Build history of the part. All positions in model axes, mm. A direction names the side the tool comes from. Coordinates: 2 decimals unless noted, no trailing zeros. Loops run counter-clockwise (first coordinate to the right, second up) from the corner with the lowest first, then second, coordinate; pieces in that order, holes last.
(1) Wall check: L1, parallel to Y at x = -120, z = 8.25; L2, parallel to X at y = -18, z = 8.5; L3, parallel to X at y = -18.5, z = 6.5. Give the ranges that are in metal, low to high.
(2) Slice it at D-D (x = 73). Give the cut face in (y, z), and give its area (3 significant figures).
(3) Slice it at B-B (z = 7). Give the number of separate pieces and of enclosed holes in the cut face, and give its area (3 significant figures).
(4) Flat gauge pins, fed straight in: P1, Ø5, axis at x = -32.04, y = -18.5, coming from the -Z side; P2, Ø1.9, axis at x = -97.09, y = 54.66, coming from the +Z side. Where does each tip first touch, or does it go through?
(5) Slice it at C-C (x = -49.5). Give the cut face in (y, z).
(6) Slice it at A-A (x = 8.5). Give the cut face in (y, z).
(7) Two-plate mould, pull along X, no slides. Class faces 1 (the face through (-150, -2, 5)), 2 (the face through (2, -150, 5)), 3 (the face through (1, -39, 3)): pulls with the +X half, pulls with the -X half, needs draft (parallel to the pull), parting line crosses it, or undercut.
(8) Tool access for faces 4 (the face through (-41.53, -79.845, 1.479)), 5 (the face through (-2, 150, 5)): list every direction of +Z, -Z, +X, -X, +Y, -Y with a clear straight run to the whole face (end or side of a thin tool).
Autodesk Inventor part; units mm, degrees
ref_plane "YZ Plane" through (0, 0, 0) normal (1, 0, 0) x (0, 1, 0)
ref_plane "XZ Plane" through (0, 0, 0) normal (0, 1, 0) x (-1, 0, 0)
ref_plane "XY Plane" through (0, 0, 0) normal (0, 0, 1) x (1, 0, 0)
sketch "スケッチ1" plane through (-150, -150, 0) normal (0, 0, 1) x (1, 0, 0)
  circle A0 centre (59.9853, 240.0147) radius 24 construction
  circle A1 centre (59.9853, 240.0147) radius 24 construction
  circle A2 centre (84.0269, 264.0563) radius 10 construction
  line L0 (84.0269, 264.0563) -> (59.9853, 240.0147) construction
  line L1 (59.9853, 240.0147) -> (84.0269, 215.9731) construction
  arc A3 (84.5273, 253.0677) -> (73.0383, 264.5567) centre (84.0269, 264.0563) ccw
  arc A4 (70.2215, 262.823) -> (82.7936, 250.2509) centre (59.9853, 240.0147) ccw
  arc A5 (84.5273, 253.0677) -> (82.7936, 250.2509) centre (84.6183, 251.0698) ccw
  arc A6 (70.2215, 262.823) -> (73.0383, 264.5567) centre (71.0404, 264.6477) ccw
  line L2 (67.0564, 275.37) -> (24.63, 232.9436) construction
  line L3 (24.63, 232.9436) -> (52.9142, 204.6594) construction
  line L4 (52.9142, 204.6594) -> (95.3406, 247.0858) construction
  line L5 (95.3406, 247.0858) -> (67.0564, 275.37) construction
  line L6 (67.0564, 275.37) -> (52.9142, 204.6594) construction
  line L7 (24.63, 232.9436) -> (95.3406, 247.0858) construction
  circle A7 centre (95.3406, 247.0858) radius 1.6
  circle A8 centre (52.9142, 204.6594) radius 1.6
  circle A9 centre (24.63, 232.9436) radius 1.6
  circle A10 centre (67.0564, 275.37) radius 1.6
  line L8 (270, 30) -> (30, 30) construction
  line L9 (30, 30) -> (30, 270) construction
  line L10 (30, 270) -> (270, 270) construction
  line L11 (270, 270) -> (270, 30) construction
  line L12 (270, 30) -> (30, 270) construction
  line L13 (30, 30) -> (270, 270) construction
  circle A11 centre (30, 270) radius 2
  circle A12 centre (270, 270) radius 2
  circle A13 centre (30, 30) radius 2
  circle A14 centre (270, 30) radius 2
  circle A15 centre (150, 150) radius 30
  line L14 (150, 113) -> (117.9571, 131.5) construction
  line L15 (117.9571, 131.5) -> (117.9571, 168.5) construction
  line L16 (117.9571, 168.5) -> (150, 187) construction
  line L17 (150, 187) -> (182.0429, 168.5) construction
  line L18 (182.0429, 168.5) -> (182.0429, 131.5) construction
  line L19 (182.0429, 131.5) -> (150, 113) construction
  circle A16 centre (150, 150) radius 37 construction
  circle A17 centre (150, 113) radius 1.6
  circle A18 centre (54.1207, 93.2509) radius 1.6 construction
  line L20 (117.9571, 131.5) -> (117.9571, 168.5) construction
  line L21 (150, 113) -> (117.9571, 131.5) construction
  line L22 (117.9571, 168.5) -> (150, 187) construction
  line L23 (182.0429, 131.5) -> (150, 113) construction
  circle A19 centre (150, 150) radius 30 construction
  line L24 (150, 187) -> (182.0429, 168.5) construction
  line L25 (182.0429, 168.5) -> (182.0429, 131.5) construction
  circle A20 centre (150, 150) radius 37 construction
  circle A21 centre (182.0429, 131.5) radius 1.6
  circle A22 centre (151.2065, 38.5916) radius 1.6 construction
  line L26 (150, 113) -> (117.9571, 131.5) construction
  line L27 (182.0429, 131.5) -> (150, 113) construction
  line L28 (117.9571, 131.5) -> (117.9571, 168.5) construction
  line L29 (182.0429, 168.5) -> (182.0429, 131.5) construction
  circle A23 centre (150, 150) radius 30 construction
  line L30 (117.9571, 168.5) -> (150, 187) construction
  line L31 (150, 187) -> (182.0429, 168.5) construction
  circle A24 centre (150, 150) radius 37 construction
  circle A25 centre (182.0429, 168.5) radius 1.6
  circle A26 centre (247.0858, 95.3406) radius 1.6 construction
  line L32 (182.0429, 131.5) -> (150, 113) construction
  line L33 (182.0429, 168.5) -> (182.0429, 131.5) construction
  line L34 (150, 113) -> (117.9571, 131.5) construction
  line L35 (150, 187) -> (182.0429, 168.5) construction
  circle A27 centre (150, 150) radius 30 construction
  line L36 (117.9571, 131.5) -> (117.9571, 168.5) construction
  line L37 (117.9571, 168.5) -> (150, 187) construction
  circle A28 centre (150, 150) radius 37 construction
  circle A29 centre (150, 187) radius 1.6
  circle A30 centre (245.8793, 206.7491) radius 1.6 construction
  line L38 (182.0429, 168.5) -> (182.0429, 131.5) construction
  line L39 (150, 187) -> (182.0429, 168.5) construction
  line L40 (182.0429, 131.5) -> (150, 113) construction
  line L41 (117.9571, 168.5) -> (150, 187) construction
  circle A31 centre (150, 150) radius 30 construction
  line L42 (150, 113) -> (117.9571, 131.5) construction
  line L43 (117.9571, 131.5) -> (117.9571, 168.5) construction
  circle A32 centre (150, 150) radius 37 construction
  circle A33 centre (117.9571, 168.5) radius 1.6
  circle A34 centre (148.7935, 261.4084) radius 1.6 construction
  line L44 (150, 187) -> (182.0429, 168.5) construction
  line L45 (117.9571, 168.5) -> (150, 187) construction
  line L46 (182.0429, 168.5) -> (182.0429, 131.5) construction
  line L47 (117.9571, 131.5) -> (117.9571, 168.5) construction
  circle A35 centre (150, 150) radius 30 construction
  line L48 (182.0429, 131.5) -> (150, 113) construction
  line L49 (150, 113) -> (117.9571, 131.5) construction
  circle A36 centre (150, 150) radius 37 construction
  circle A37 centre (117.9571, 131.5) radius 1.6
  line L50 (0, 300) -> (300, 300)
  line L51 (300, 300) -> (300, 0)
  line L52 (300, 0) -> (0, 0)
  line L53 (0, 0) -> (0, 300)
  line L54 (0, 300) -> (300, 0) construction
  line L55 (300, 300) -> (0, 0) construction
  point P0 (150, 150)
  point P1 (81.1985, 261.2279)
  point P2 (150, 150)
  point P3 (59.8791, 125.8522)
  point P4 (150, 150)
  point P5 (125.8522, 59.8791)
  point P6 (150, 150)
  point P7 (215.9731, 84.0269)
  point P8 (150, 150)
  point P9 (240.1209, 174.1478)
  point P10 (150, 150)
  point P11 (174.1478, 240.1209)
  dimension "d30" = 74
  dimension "d6" = 48
  dimension "d7" = 20
  dimension "d10" = 25
  dimension "d11" = 11
  dimension "d12" = 2
  dimension "d15" = 40
  dimension "d16" = 60
  dimension "d17" = 3.2
  dimension "d18" = 240
  dimension "d19" = 4
  dimension "d22" = 240
  dimension "d25" = 240
  dimension "d28" = 60
  dimension "d31" = 3.2
  dimension "d34" = 360
  dimension "d36" = 300
  dimension "d39" = 127.3
  dimension "d40" = 3.2
  dimension "d41" = 48
extrude "押し出し2" add sketch "スケッチ1" along normal blind 10
sketch "スケッチ2" plane through (-150, -150, 0) normal (0, 0, -1) x (-1, 0, 0)
  circle A0 centre (-150, 150) radius 90
  dimension "d42" = 180
extrude "押し出し3" cut sketch "スケッチ2" against normal blind 3
properties part number "ロボットベース2019" material "マツ材"
Response values:
1. L1: y = -150 to -122, -118 to 118, 122 to 150
1. L2: x = -150 to -33.56, -30.52 to -24, 24 to 30.52, 33.56 to 150
1. L3: x = -150 to -33.64, -30.44 to -23.62, 23.62 to 30.44, 33.64 to 150
2. outline: (-150, 0) - (-52.64, 0) - (-52.64, 3) - (52.64, 3) - (52.64, 0) - (150, 0) - (150, 10) - (-150, 10) - close
2. area: 2,680 mm2
3. separate pieces: 1
3. enclosed holes: 16
3. area: 84,700 mm2
4. P1: stops at z = 3
4. P2: passes through
5. outline: (-150, 0) - (-75.16, 0) - (-75.16, 3) - (75.16, 3) - (75.16, 0) - (150, 0) - (150, 10) - (-150, 10) - close
6. outline: (-150, 0) - (-89.6, 0) - (-89.6, 3) - (-28.77, 3) - (-28.77, 10) - (-150, 10) - close; (28.77, 3) - (89.6, 3) - (89.6, 0) - (150, 0) - (150, 10) - (28.77, 10) - close
7. face 1: pulls with the -X half
7. face 2: needs draft
7. face 3: undercut
8. face 4: -Z
8. face 5: +Z, -Z, +X, -X, +Y
